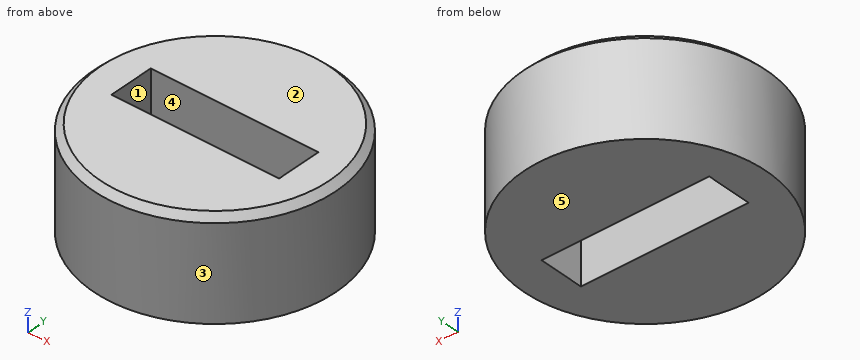
from build123d import *

# Parameters (mm, degrees)
F0_R     = 92.15231
F1_DEPTH = 76.2
F2_SIZE  = 5.08
F3_W     = 127.593874
F3_H     = 34.602892
F4_DEPTH = 115.57


with BuildPart() as f1:
    # F0 (on Top) → F1 (new body)
    with BuildSketch(Plane.XY):
        Circle(F0_R)
    extrude(amount=F1_DEPTH)

    # F2
    f2_edges = [f1.edges().sort_by_distance(p)[0] for p in [
        (-92.15231, 0, 76.2),
    ]]
    chamfer(f2_edges, length=F2_SIZE)

    # F3 (on face) → F4 (cut)
    with BuildSketch(Plane.XY.offset(76.2)):
        Rectangle(F3_W, F3_H)
    extrude(amount=-F4_DEPTH, mode=Mode.SUBTRACT)


solid = f1.part
Geometry: final body of the model. Coordinates: model frame, mm. Face numbers are marked on the shaded views. A direction names the side the tool comes from. Give positions to 0.01 mm unless a question says otherwise; leave off trailing zeros. Loops run counter-clockwise (first coordinate to the right, second up) from the corner with the lowest first, then second, coordinate; pieces in that order, holes last. Notation, with made-up numbers: (-4.75, 67) -> (46.25, 67) arc R9 ccw to (46.25, 76) -> close; hole circle Ø3 at (-35.5, 36). An arc over 180 degrees is marked (long way). Put each result on its own line as item: value.
1. Ray query, line 1 along Y through (x, z) = (31, 24); line 2 along X through (y, z) = (11, 46.5); line 3 along X through (y, z) = (-9, 52.5). Return the intervals inside material, ascending. Write a range as [from, to].
Taken from the geometry:
line 1: y = [-86.78, -17.3], [17.3, 86.78]
line 2: x = [-91.49, -63.8], [63.8, 91.49]
line 3: x = [-91.71, -63.8], [63.8, 91.71]
2. Cut plane B-B (z = 28). Return the cut outline in (x, y).
Taken from the geometry:
outline: circle Ø184.3 at (0, 0); hole (-63.8, -17.3) -> (63.8, -17.3) -> (63.8, 17.3) -> (-63.8, 17.3) -> close
3. Pin query (flat end, axial travel): P1, Ø6, axis at y = -47, z = 20.5, coming from the -X side; P2, Ø4, axis at y = 51, z = 66.5, coming from the -X side; P3, Ø5, axis at y = -51, z = 65.5, coming from the -X side. Return the tip coordinate at first contact, or that it passes through.
Taken from the geometry:
P1: stops at x = -80.97
P2: stops at x = -78.05
P3: stops at x = -78.36
4. Set-up query: the marked faces 1 and 2. Return all of +Z, -Z, +X, -X, +Y, -Y with unobstructed straight access to the full face (end or side cutting, diameter ignored); none if empty.
Taken from the geometry:
face 1: +Z, -Z
face 2: +Z, +X, -X, +Y, -Y
5. Cut plane A-A (x = 0). Return the cut outline in (y, z).
Taken from the geometry:
outline: (-92.15, 0) -> (-17.3, 0) -> (-17.3, 76.2) -> (-87.07, 76.2) -> (-92.15, 71.12) -> close; (17.3, 0) -> (92.15, 0) -> (92.15, 71.12) -> (87.07, 76.2) -> (17.3, 76.2) -> close
6. Cut plane C-C (y = 0). Return the cut outline in (x, z), plus the area to 3 significant figures.
Taken from the geometry:
outline: (-92.15, 0) -> (-63.8, 0) -> (-63.8, 76.2) -> (-87.07, 76.2) -> (-92.15, 71.12) -> close; (63.8, 0) -> (92.15, 0) -> (92.15, 71.12) -> (87.07, 76.2) -> (63.8, 76.2) -> close
area: 4,300 mm2
7. Pull-direction query (Y, two-part tool) for the marked faces 3, 4 and 5; classes: released by +Y, released by -Y, zero draft, split by the parting line, or undercut.
Taken from the geometry:
face 3: split by the parting line
face 4: undercut
face 5: zero draft
